Could you check a few things on this model? Use its own coordinates, in mm. Round coordinates to 2 decimals unless told otherwise and drop trailing zeros. Loops run counter-clockwise (first coordinate to the right, second up) from the corner with the lowest first, then second, coordinate; pieces in that order, holes last. Notation, with made-up numbers: M 81.25,76.25 L 88.25,76.25 A25 ccw 88.25,98.25 Z; hole C 58.25,-5.75 d10. An arc over 180 degrees is marked long. Answer in a Markdown table with one row per item.
```python
from build123d import *

# Parameters (mm, degrees)
SKETCH1_R                       = 5
BOSS_EXTRUDE1_DEPTH             = 100
CUT_EXTRUDE5_REACH              = 7
SKETCH2_W                       = 3
SKETCH2_H                       = 11
CUT_EXTRUDE5_DIRECTION_2_REACH  = 7
CUT_EXTRUDE6_REACH              = 9
SKETCH3_R                       = 2.5
M6X1_0_TAPPED_HOLE1_D           = 5
M6X1_0_TAPPED_HOLE1_DEPTH       = 17
M6X1_0_TAPPED_HOLE1_CSINK_D     = 6.5
M6X1_0_TAPPED_HOLE1_CSINK_ANGLE = 90
M6X1_0_TAPPED_HOLE1_TIP         = 1.502151548


with BuildPart() as part:
    # Sketch1 → Boss-Extrude1 (new body)
    with BuildSketch(Plane.XY):
        Circle(SKETCH1_R)
    extrude(amount=-BOSS_EXTRUDE1_DEPTH)

    # Sketch2 → Cut-Extrude5 (cut, up to next)
    with BuildSketch(Plane(origin=(0, 0, 0), x_dir=(1, 0, 0), z_dir=(0, 1, 0)), mode=Mode.PRIVATE) as cut_extrude5_sk1:
        with Locations((-3.5, 94.5)):
            Rectangle(SKETCH2_W, SKETCH2_H)
    cut_extrude5_tool1 = extrude(cut_extrude5_sk1.sketch, amount=-CUT_EXTRUDE5_REACH, mode=Mode.PRIVATE) & part.part
    add(cut_extrude5_tool1.solids().sort_by_distance((-3.5, 0, -94.5))[0], mode=Mode.SUBTRACT)
    # Sketch2 → Cut-Extrude5 (cut, up to next)
    with BuildSketch(Plane(origin=(0, 0, 0), x_dir=(1, 0, 0), z_dir=(0, 1, 0)), mode=Mode.PRIVATE) as cut_extrude5_sk2:
        with Locations((3.5, 94.5)):
            Rectangle(SKETCH2_W, SKETCH2_H)
    cut_extrude5_tool2 = extrude(cut_extrude5_sk2.sketch, amount=-CUT_EXTRUDE5_REACH, mode=Mode.PRIVATE) & part.part
    add(cut_extrude5_tool2.solids().sort_by_distance((3.5, 0, -94.5))[0], mode=Mode.SUBTRACT)

    # Sketch2 → Cut-Extrude5 direction 2 (cut, up to next)
    with BuildSketch(Plane(origin=(0, 0, 0), x_dir=(1, 0, 0), z_dir=(0, 1, 0)), mode=Mode.PRIVATE) as cut_extrude5_direction_2_sk1:
        with Locations((-3.5, 94.5)):
            Rectangle(SKETCH2_W, SKETCH2_H)
    cut_extrude5_direction_2_tool1 = extrude(cut_extrude5_direction_2_sk1.sketch, amount=CUT_EXTRUDE5_DIRECTION_2_REACH, mode=Mode.PRIVATE) & part.part
    add(cut_extrude5_direction_2_tool1.solids().sort_by_distance((-3.5, 0, -94.5))[0], mode=Mode.SUBTRACT)
    # Sketch2 → Cut-Extrude5 direction 2 (cut, up to next)
    with BuildSketch(Plane(origin=(0, 0, 0), x_dir=(1, 0, 0), z_dir=(0, 1, 0)), mode=Mode.PRIVATE) as cut_extrude5_direction_2_sk2:
        with Locations((3.5, 94.5)):
            Rectangle(SKETCH2_W, SKETCH2_H)
    cut_extrude5_direction_2_tool2 = extrude(cut_extrude5_direction_2_sk2.sketch, amount=CUT_EXTRUDE5_DIRECTION_2_REACH, mode=Mode.PRIVATE) & part.part
    add(cut_extrude5_direction_2_tool2.solids().sort_by_distance((3.5, 0, -94.5))[0], mode=Mode.SUBTRACT)

    # Sketch3 → Cut-Extrude6 (cut, up to next)
    with BuildSketch(Plane(origin=(2, 0, 0), x_dir=(0, 0, -1), z_dir=(1, 0, 0)), mode=Mode.PRIVATE) as cut_extrude6_sk1:
        with Locations((95, 0)):
            Circle(SKETCH3_R)
    cut_extrude6_tool1 = extrude(cut_extrude6_sk1.sketch, amount=-CUT_EXTRUDE6_REACH, mode=Mode.PRIVATE) & part.part
    add(cut_extrude6_tool1.solids().sort_by_distance((2, 0, -95))[0], mode=Mode.SUBTRACT)

    # M6x1.0 Tapped Hole1
    with Locations(Plane.XY):
        with Locations((0, 0)):
            CounterSinkHole(M6X1_0_TAPPED_HOLE1_D / 2, M6X1_0_TAPPED_HOLE1_CSINK_D / 2, depth=M6X1_0_TAPPED_HOLE1_DEPTH, counter_sink_angle=M6X1_0_TAPPED_HOLE1_CSINK_ANGLE)
            with Locations((0, 0, -(M6X1_0_TAPPED_HOLE1_DEPTH + M6X1_0_TAPPED_HOLE1_TIP / 2))):  # 118° drill point
                Cone(0, M6X1_0_TAPPED_HOLE1_D / 2, M6X1_0_TAPPED_HOLE1_TIP, mode=Mode.SUBTRACT)


solid = part.part
```
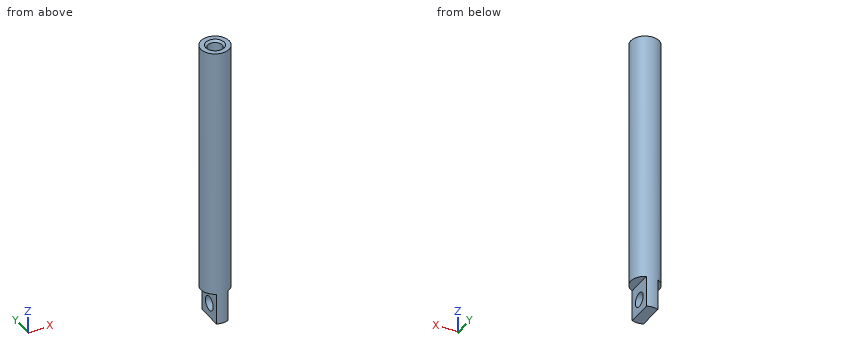
1) I want a section at A-A, the plane z = -95. Please give me the cut outline in (x, y).
Computed:
| item | result |
|---|---|
| outline | M -2,-4.58 A5 ccw 2,-4.58 L 2,-2.5 L -2,-2.5 Z; M -2,2.5 L 2,2.5 L 2,4.58 A5 ccw -2,4.58 Z |
2) Will these pins go through, and if not, where does the flat tip stop? P1, Ø3, axis at x = -0.5, z = -33, coming from the +Y side; P2, Ø2.5, axis at y = 0.5, z = -92, coming from the +X side; P3, Ø2.5, axis at y = -2, z = -95.5, coming from the -X side; P4, Ø5, axis at y = 4, z = -49, coming from the +X side.
Computed:
| item | result |
|---|---|
| P1 | stops at y = 5 |
| P2 | stops at x = 2 |
| P3 | stops at x = -2 |
| P4 | stops at x = 4.77 |
3) I need wall thicknesses on line 1 (Y direction, x = 0, z = -8.5); line 2 (Z direction, x = 2.5, y = -3.75); line 3 (Z direction, x = 1.75, y = 1.25). Which ranges of each line are inside material? Lowest first, please.
Computed:
| item | result |
|---|---|
| line 1 | y = -5 to -2.5, 2.5 to 5 |
| line 2 | z = -89 to 0 |
| line 3 | z = -100 to -97.17, -92.83 to -17.21 |
4) I want a section at B-B, the plane z = -8. Please give me the cut outline in (x, y).
Computed:
| item | result |
|---|---|
| outline | C 0,0 d10; hole C 0,0 d5 |
